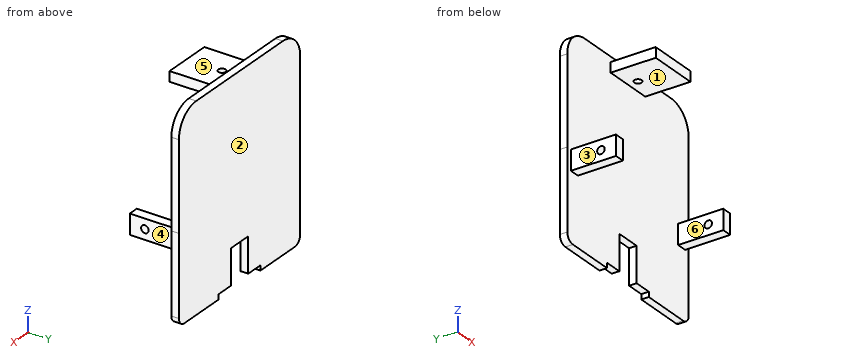
from build123d import *

# Parameters (mm, degrees)
BOSS_EXTRUDE4_DEPTH    = 0.75
EXTRUDE_THIN2_DEPTH    = 0.75
UPPER_17_W             = 5
UPPER_17_H             = 1
UPPER_17_W_2           = 1
UPPER_17_H_2           = 2
LID_ANCHOR_FRONT_DEPTH = 4.5
TAP_LATERAL_LID_D      = 0.75
TAP_FRONT_LID_D        = 0.75
CUT_EXTRUDE1_REACH     = 16.029


with BuildPart() as part:
    # upper_13 → Boss-Extrude4 (new body)
    with BuildSketch(Plane(origin=(0, -19, 0), x_dir=(1, 0, 0), z_dir=(0, 1, 0))):
        with BuildLine():
            Line((-6.250353693, -9.5), (6.250353693, -9.5))
            ThreePointArc((6.250353693, -9.5), (7.665029054, -8.913751613), (8.250353267, -7.498693623))
            ThreePointArc((8.250353267, -7.498693623), (8.248836313, -3.124346866), (8.25, 1.25))
            Line((8.25, 1.25), (8.25, 9.2))
            ThreePointArc((8.25, 9.2), (8.162132034, 9.412132034), (7.95, 9.5))
            Line((7.95, 9.5), (1.25, 9.5))
            Line((1.25, 9.5), (1.25, 6))
            Line((1.25, 6), (-1.25, 6))
            Line((-1.25, 6), (-1.25, 9.5))
            Line((-1.25, 9.5), (-7.95, 9.5))
            ThreePointArc((-7.95, 9.5), (-8.162132034, 9.412132034), (-8.25, 9.2))
            Line((-8.25, 9.2), (-8.25, 1.25))
            ThreePointArc((-8.25, 1.25), (-8.199296345, -3.106194095), (-8.25, -7.462388189))
            ThreePointArc((-8.25, -7.462388189), (-7.677803101, -8.900852665), (-6.250353693, -9.5))
        make_face()
    extrude(amount=BOSS_EXTRUDE4_DEPTH)



with BuildPart() as body_2:
    # upper_16 → Extrude-Thin2 (new body)
    with BuildSketch(Plane(origin=(0, -19, 0), x_dir=(1, 0, 0), z_dir=(0, 1, 0))):
        with BuildLine():
            Line((-8.75, 1.244176388), (-8.75, 9.2))
            ThreePointArc((-8.75, 9.2), (-8.515685425, 9.765685425), (-7.95, 10))
            Line((-7.95, 10), (7.95, 10))
            ThreePointArc((7.95, 10), (8.515685425, 9.765685425), (8.75, 9.2))
            Line((8.75, 9.2), (8.75, 1.24985689))
            ThreePointArc((8.75, 1.24985689), (8.74883631, -3.124255124), (8.75035316, -7.498367029))
            ThreePointArc((8.75035316, -7.498367029), (8.018697895, -9.267189516), (6.250353693, -10))
            Line((6.250353693, -10), (-6.250353693, -10))
            ThreePointArc((-6.250353693, -10), (-8.035078913, -9.250644422), (-8.749889093, -7.451804713))
            ThreePointArc((-8.749889093, -7.451804713), (-8.69929636, -3.103813517), (-8.75, 1.244176388))
        make_face()
        with BuildLine():
            Line((-8.25, 1.25), (-8.25, 9.2))
            ThreePointArc((-8.25, 9.2), (-8.162132034, 9.412132034), (-7.95, 9.5))
            Line((-7.95, 9.5), (7.95, 9.5))
            ThreePointArc((7.95, 9.5), (8.162132034, 9.412132034), (8.25, 9.2))
            Line((8.25, 9.2), (8.25, 1.25))
            ThreePointArc((8.25, 1.25), (8.248836313, -3.124346866), (8.250353267, -7.498693623))
            ThreePointArc((8.250353267, -7.498693623), (7.665029054, -8.913751613), (6.250353693, -9.5))
            Line((6.250353693, -9.5), (-6.250353693, -9.5))
            ThreePointArc((-6.250353693, -9.5), (-7.677803101, -8.900852665), (-8.25, -7.462388189))
            ThreePointArc((-8.25, -7.462388189), (-8.199296345, -3.106194095), (-8.25, 1.25))
        make_face(mode=Mode.SUBTRACT)
    extrude(amount=EXTRUDE_THIN2_DEPTH)


with BuildPart() as part_1:
    add(part.part)

    add(body_2.part)  # lid_anchor_front merges body 2
    # upper_17 → lid_anchor_front (add)
    with BuildSketch(Plane(origin=(0, -19, 0), x_dir=(1, 0, 0), z_dir=(0, 1, 0))):
        with Locations((0, -8.99)):
            Rectangle(UPPER_17_W, UPPER_17_H)
        with Locations((-7.74, 2.25)):
            Rectangle(UPPER_17_W_2, UPPER_17_H_2)
    lid_anchor_front = extrude(amount=-LID_ANCHOR_FRONT_DEPTH)

    # tap_lateral_lid (through all)
    with Locations(Plane.ZY.offset(8.24)):
        with Locations((-2.25, -22)):
            tap_lateral_lid = Hole(TAP_LATERAL_LID_D / 2)

    # Mirror3: lid_anchor_front, tap_lateral_lid across plane
    add(lid_anchor_front.mirror(Plane(origin=(0, 0, 0), x_dir=(0, 0, 1), z_dir=(1, 0, 0))))
    add(tap_lateral_lid.mirror(Plane(origin=(0, 0, 0), x_dir=(0, 0, 1), z_dir=(1, 0, 0))), mode=Mode.SUBTRACT)

    # tap_front_lid (through all)
    with Locations(Plane.XY.offset(9.49)):
        with Locations((0, -20)):
            Hole(TAP_FRONT_LID_D / 2)

    # upper_18 → Cut-Extrude1 (cut, up to next)
    with BuildSketch(Plane(origin=(0, -19, 0), x_dir=(1, 0, 0), z_dir=(0, 1, 0)), mode=Mode.PRIVATE) as cut_extrude1_sk1:
        with BuildLine():
            ThreePointArc((-2.5, 9.5), (-1.767766953, 11.267766953), (0, 12))
            Line((0, 12), (-1.556624327, 12))
            Line((-1.556624327, 12), (-3, 9.5))
            Line((-3, 9.5), (-2.5, 9.5))
        make_face()
    cut_extrude1_tool1 = extrude(cut_extrude1_sk1.sketch, amount=CUT_EXTRUDE1_REACH, mode=Mode.PRIVATE) & part_1.part
    # upper_18 → Cut-Extrude1 (cut, up to next)
    with BuildSketch(Plane(origin=(0, -19, 0), x_dir=(1, 0, 0), z_dir=(0, 1, 0)), mode=Mode.PRIVATE) as cut_extrude1_sk2:
        with BuildLine():
            Line((2.5, 9.5), (3, 9.5))
            Line((3, 9.5), (1.556624327, 12))
            Line((1.556624327, 12), (0, 12))
            ThreePointArc((0, 12), (1.767766953, 11.267766953), (2.5, 9.5))
        make_face()
    cut_extrude1_tool2 = extrude(cut_extrude1_sk2.sketch, amount=CUT_EXTRUDE1_REACH, mode=Mode.PRIVATE) & part_1.part
    # upper_18 → Cut-Extrude1 (cut, up to next)
    with BuildSketch(Plane(origin=(0, -19, 0), x_dir=(1, 0, 0), z_dir=(0, 1, 0)), mode=Mode.PRIVATE) as cut_extrude1_sk3:
        with BuildLine():
            Line((1.25, 9.5), (2.5, 9.5))
            ThreePointArc((2.5, 9.5), (1.767766953, 11.267766953), (0, 12))
            ThreePointArc((0, 12), (-1.767766953, 11.267766953), (-2.5, 9.5))
            Line((-2.5, 9.5), (-1.25, 9.5))
            Line((-1.25, 9.5), (1.25, 9.5))
        make_face()
    cut_extrude1_tool3 = extrude(cut_extrude1_sk3.sketch, amount=CUT_EXTRUDE1_REACH, mode=Mode.PRIVATE) & part_1.part
    # upper_18 → Cut-Extrude1 (cut, up to next)
    with BuildSketch(Plane(origin=(0, -19, 0), x_dir=(1, 0, 0), z_dir=(0, 1, 0)), mode=Mode.PRIVATE) as cut_extrude1_sk4:
        Polygon((1.556624327, 12), (3, 9.5), (3, 12), align=None)
    cut_extrude1_tool4 = extrude(cut_extrude1_sk4.sketch, amount=CUT_EXTRUDE1_REACH, mode=Mode.PRIVATE) & part_1.part
    # upper_18 → Cut-Extrude1 (cut, up to next)
    with BuildSketch(Plane(origin=(0, -19, 0), x_dir=(1, 0, 0), z_dir=(0, 1, 0)), mode=Mode.PRIVATE) as cut_extrude1_sk5:
        Polygon((-3.025026025, 12), (-3.025026025, 9.5), (-3, 9.5), (-1.556624327, 12), align=None)
    cut_extrude1_tool5 = extrude(cut_extrude1_sk5.sketch, amount=CUT_EXTRUDE1_REACH, mode=Mode.PRIVATE) & part_1.part
    add(cut_extrude1_tool1.solids().sort_by_distance((-2.75, -19, -9.539051))[0], mode=Mode.SUBTRACT)
    add(cut_extrude1_tool2.solids().sort_by_distance((2.244493, -19, -10.730474))[0], mode=Mode.SUBTRACT)
    add(cut_extrude1_tool3.solids().sort_by_distance((0, -19, -10.561033))[0], mode=Mode.SUBTRACT)
    add(cut_extrude1_tool4.solids().sort_by_distance((2.518875, -19, -11.166667))[0], mode=Mode.SUBTRACT)
    add(cut_extrude1_tool5.solids().sort_by_distance((-2.535419, -19, -11.152702))[0], mode=Mode.SUBTRACT)


solid = part_1.part
Model file for the job. Use its own axes, mm. Face numbers are marked on the shaded views. A direction names the side the tool comes from. Coordinates: 2 decimals unless noted, no trailing zeros. Write each loop counter-clockwise with the first axis right and the second up, starting at its lowest first coordinate (ties: lowest second). Pieces come first, ordered by that corner, then holes. Notation, with made-up numbers: (-30, -26) -> (9, -26) arc R19 ccw to (9, -8) -> close; hole circle Ø7 at (57.5, 10). An arc over 180 degrees is marked (long way). One line per item, written item: value. Start each with the question number.
1) Probe probe 1 along X at (y, z) = (-21, -2.75); probe 2 along Z at (x, y) = (-7.8, -22) (3 decimals); probe 3 along X at (y, z) = (-20, 9.15) (3 decimals). List the from-to ranges inside material, lowest first.
2) Pull direction X, two halves, no side cores. Call the marked faces 4, 5 and 6: +X half, -X half, draft (parallel to the pull), parting line (faces both ways), or undercut.
3) Slice it at D-D on z = -7.75. Write the cut outline in (x, y), then the cut area to 4 significant figures.
4) Slice it at A-A on y = -22. Write the cut outline in (x, z) (3 decimals), then the cut area to 3 significant figures.
5) Flat gauge pins, fed straight in: pin 1 Ø1.1 at (x, y) = (8, -20.5) entering from -Z; pin 2 Ø10 at (x, z) = (-0.5, -2.5) entering from -Y; pin 3 Ø1.1 at (x, y) = (-7.5, -21) entering from +Z; pin 4 Ø1 at (y, z) = (-22, 7.5) entering from -X. Where does each tip first touch, or does it go through?
6) Slice it at B-B on z = -2.25. Write the cut outline in (x, y) (3 decimals).
7) Slice it at C-C on x = 0. Write the cut outline in (y, z) (3 decimals), then the cut area to 4 significant figures.
8) Which spindle directions (+Z, -Z, +X, -X, +Y, -Y) get a long thin tool onto all of the face, cutting with end or side? Do the marked faces 1, 2 and 3. Say none if no direction does.
Answers follow:
1. probe 1: -8.24 to -7.24, 7.24 to 8.24
1. probe 2: -3.25 to -2.625, -1.875 to -1.25
1. probe 3: -2.5 to -0.375, 0.375 to 2.5
2. face 4: +X half
2. face 5: draft
2. face 6: undercut
3. outline: (-8.75, -19) -> (-1.25, -19) -> (-1.25, -18.25) -> (-8.75, -18.25) -> close; (1.25, -19) -> (8.75, -19) -> (8.75, -18.25) -> (1.25, -18.25) -> close
3. area: 11.25 mm2
4. outline: (-8.24, -3.25) -> (-7.24, -3.25) -> (-7.24, -2.625) -> (-8.24, -2.625) -> close; (-8.24, -1.875) -> (-7.24, -1.875) -> (-7.24, -1.25) -> (-8.24, -1.25) -> close; (-2.5, 8.49) -> (2.5, 8.49) -> (2.5, 9.49) -> (-2.5, 9.49) -> close; (7.24, -3.25) -> (8.24, -3.25) -> (8.24, -2.625) -> (7.24, -2.625) -> close; (7.24, -1.875) -> (8.24, -1.875) -> (8.24, -1.25) -> (7.24, -1.25) -> close
4. area: 7.50 mm2
5. pin 1: z = -3.25
5. pin 2: y = -19
5. pin 3: z = -1.25
5. pin 4: through
6. outline: (-8.75, -19) -> (-8.24, -19) -> (-8.24, -21.625) -> (-7.24, -21.625) -> (-7.24, -19) -> (7.24, -19) -> (7.24, -21.625) -> (8.24, -21.625) -> (8.24, -19) -> (8.75, -19) -> (8.75, -18.25) -> (-8.75, -18.25) -> close; (-8.24, -23.5) -> (-7.24, -23.5) -> (-7.24, -22.375) -> (-8.24, -22.375) -> close; (7.24, -23.5) -> (8.24, -23.5) -> (8.24, -22.375) -> (7.24, -22.375) -> close
7. outline: (-23.5, 8.49) -> (-20.375, 8.49) -> (-20.375, 9.49) -> (-23.5, 9.49) -> close; (-19.625, 8.49) -> (-19, 8.49) -> (-19, -6) -> (-18.25, -6) -> (-18.25, 10) -> (-19, 10) -> (-19, 9.49) -> (-19.625, 9.49) -> close
7. area: 15.75 mm2
8. face 1: -Z, +X, -X, -Y
8. face 2: +Z, -Z, +X, -X, +Y
8. face 3: +Z, -Z, -X, -Y
